Can you work these out from the model? Positions are in its coordinate system, mm. A direction names the side the tool comes from. Give positions to 0.01 mm unless a question says otherwise; leave off trailing zeros. Loops run counter-clockwise (first coordinate to the right, second up) from the corner with the lowest first, then second, coordinate; pieces in that order, holes last. Notation, with made-up numbers: (-26.75, 13.5) - (22.25, 13.5) arc R25 cw to (22.25, 27.5) - close; hole circle Ø2 at (72.5, 60). An arc over 180 degrees is marked (long way). Answer as a JSON object with one key per item and string values.
Autodesk Inventor part; units mm, degrees
ref_plane "YZ Plane" through (0, 0, 0) normal (1, 0, 0) x (0, 1, 0)
ref_plane "XZ Plane" through (0, 0, 0) normal (0, 1, 0) x (-1, 0, 0)
ref_plane "XY Plane" through (0, 0, 0) normal (0, 0, 1) x (1, 0, 0)
sketch "Sketch1" plane through (0, 0, 0) normal (0, 1, 0) x (-1, 0, 0)
  line L0 (6.7034, 26.0749) -> (-27.2966, 26.0749)
  line L1 (-32.2966, 21.0749) -> (-32.2966, -22.9251)
  line L2 (-27.2966, -27.9251) -> (6.7034, -27.9251)
  line L3 (6.7034, -27.9251) -> (6.7034, 26.0749)
  arc A0 (-27.2966, 26.0749) -> (-32.2966, 21.0749) centre (-27.2966, 21.0749) ccw
  arc A1 (-32.2966, -22.9251) -> (-27.2966, -27.9251) centre (-27.2966, -22.9251) ccw
  circle A2 centre (-22.2966, 17.0749) radius 5
  circle A3 centre (-22.2966, -18.9251) radius 5
  point P0 (0, 0)
  point P1 (-32.2966, -27.9251)
  point P2 (-32.2966, 26.0749)
  dimension "d0" = 39
  dimension "d1" = 54
  dimension "d2" = 5
  dimension "d3" = 5
  dimension "d5" = 10
  dimension "d6" = 9
  dimension "d8" = 10
  dimension "d9" = 9
extrude "Extrusion1" add sketch "Sketch1" along normal blind 8
sketch "Sketch2" plane through (0, 8, 0) normal (0, 1, 0) x (1, 0, 0)
  line L0 (-6.7034, 27.9251) -> (-6.7034, -26.0749)
  line L1 (-6.7034, -26.0749) -> (1.2966, -26.0749)
  line L2 (-6.7034, -26.0749) -> (27.2966, -26.0749)
  line L3 (1.2966, -26.0749) -> (1.2966, 27.9251)
  line L4 (1.2966, 27.9251) -> (-6.7034, 27.9251)
  line L5 (-6.7034, -26.0749) -> (-6.7034, 27.9251)
  point P0 (0, 0)
  dimension "d12" = 8
  dimension "d13" = 54
extrude "Extrusion2" cut sketch "Sketch2" against normal blind 4
ref_plane "Work Plane2" through (1.2966, 8, -27.9251) normal (-1, 0, 0) x (0, 0, 1)
sketch "Sketch3" plane through (1.2966, 8, -27.9251) normal (-1, 0, 0) x (0, 0, 1)
  line L0 (0, 0) -> (54, 0)
  circle A0 centre (27, 43) radius 5
  arc A1 (41, 43) -> (13, 43) centre (27, 43) ccw
  line L1 (13, 43) -> (13, 0)
  line L2 (4, 0) -> (14, 0)
  line L3 (41, 43) -> (41, 0)
  line L4 (13, 0) -> (41, 0)
  point P0 (27.9251, -8)
  point P1 (13, 0)
  dimension "d19" = 10
extrude "Extrusion3" add sketch "Sketch3" against normal blind 8
fillet "Fillet1" radius 5 1 edges at (5.2966, 8, -14.9251)
fillet "Fillet2" radius 5 1 edges at (5.2966, 8, 13.0749)
sketch "Sketch4" plane through (1.2966, 4, -27.9251) normal (-1, 0, 0) x (0, 0, 1)
  line L0 (0, 0) -> (0, 4)
  circle A0 centre (27, 47) radius 14
  point P0 (27.9251, -4)
extrude "Extrusion4" add sketch "Sketch4" along normal blind 8
sketch "Sketch5" plane through (-6.7034, 51, -0.9251) normal (-1, 0, 0) x (0, 0, 1)
  circle A0 centre (0, 0) radius 5
  point P0 (0.9251, -51)
  dimension "d29" = 10
extrude "Extrusion5" cut sketch "Sketch5" against normal blind 8
properties part number "4 - Part 1"
1) I'm going to push flat-ended pins straight in: P1, Ø3, axis at y = 44, z = -1, coming from the +X side; P2, Ø11.5, axis at x = 22.3, z = 17.07, coming from the +Y side; P3, Ø6.5, axis at x = 6, y = 30.5, coming from the -Z side. Where does each tip first touch, or does it pass through?
Check sheet entries:
{"P1": "x = 9.3", "P2": "y = 8", "P3": "z = -14.93"}
2) I need wall thicknesses on L1, parallel to Y at x = 1, z = -1; L2, parallel to Y at x = 22, z = -10.5; L3, parallel to X at y = 52.5, z = -14. Which ranges of each line are inside material? Lowest first, please.
Check sheet entries:
{"L1": "0 to 4, 37 to 46, 56 to 65", "L2": "0 to 8", "L3": "-6.7 to 9.3"}
3) Imagine slicing it at A-A on x = 2.5. Write out the boundary of the cut face in (y, z), and give its area (3 significant figures).
Check sheet entries:
{"outline": "(0, -27.93) - (8, -27.93) - (8, -19.93) arc R5 cw to (13, -14.93) - (51, -14.93) arc R14 ccw to (51, 13.07) - (13, 13.07) arc R5 cw to (8, 18.07) - (8, 26.07) - (0, 26.07) - close; hole circle Ø10 at (51, -0.93)", "area": "1,880 mm2"}
4) Imagine slicing it at B-B on z = -2. Write out the boundary of the cut face in (x, y), and give its area (3 significant figures).
Check sheet entries:
{"outline": "(-6.7, 0) - (32.3, 0) - (32.3, 8) - (9.3, 8) - (9.3, 46.12) - (-6.7, 46.12) - (-6.7, 37.04) - (1.3, 37.04) - (1.3, 4) - (-6.7, 4) - close; (-6.7, 55.88) - (9.3, 55.88) - (9.3, 64.96) - (-6.7, 64.96) - close", "area": "803 mm2"}
5) Which directions (+Z, -Z, +X, -X, +Y, -Y) give clear straight access to the entire face, cutting with the end or side of a thin tool? Please do faces 5 (the flat face through (9.297, 37, -1)), 6 (the flat face through (5, 32, 13.075)), 7 (the cylindrical face through (19.61, 3.94, -23.14)).
Check sheet entries:
{"face 5": "+Z, -Z, +X, +Y", "face 6": "+Z, +X, -X, +Y", "face 7": "+Y, -Y"}
6) Imagine slicing it at D-D on y = 39.5. Write out the boundary of the cut face in (x, z), and give its area (3 significant figures).
Check sheet entries:
{"outline": "(-6.7, -8.91) - (1.3, -8.91) - (1.3, -14.93) - (9.3, -14.93) - (9.3, 13.07) - (1.3, 13.07) - (1.3, 7.06) - (-6.7, 7.06) - close", "area": "352 mm2"}
7) Imagine slicing it at C-C on y = 48. Write out the boundary of the cut face in (x, z), and give its area (3 significant figures).
Check sheet entries:
{"outline": "(-6.7, -14.6) - (1.3, -14.6) - (1.3, -14.93) - (9.3, -14.93) - (9.3, -4.93) - (-6.7, -4.93) - close; (-6.7, 3.07) - (9.3, 3.07) - (9.3, 13.07) - (1.3, 13.07) - (1.3, 12.75) - (-6.7, 12.75) - close", "area": "315 mm2"}
8) If we mould it in two halves opening along Y, with no side actions, what happens to faces 1 (the flat face through (11, 4, -27.925)), 2 (the flat face through (13, 0, -1)), 3 (the flat face through (-3, 4, -1)), 4 (the cylindrical face through (-0.37, 63.42, 5.54))? For each: released by +Y, released by -Y, zero draft, split by the parting line, or undercut.
Check sheet entries:
{"face 1": "zero draft", "face 2": "released by -Y", "face 3": "undercut", "face 4": "undercut"}
